from build123d import *

# Parameters (mm, degrees)
BOSS_EXTRUDE1_DEPTH = 1.8
SKETCH2_R           = 3.25
SKETCH2_R_2         = 2.5
BOSS_EXTRUDE3_DEPTH = 0.2
SKETCH5_R           = 3.25
SKETCH5_R_2         = 2
BOSS_EXTRUDE4_DEPTH = 3
CUT_EXTRUDE1_REACH  = 6.8
SKETCH6_R           = 1.5
CUT_EXTRUDE2_REACH  = 6.8
SKETCH8_R           = 0.5


with BuildPart() as part:
    # Sketch1 → Boss-Extrude1 (new body)
    with BuildSketch(Plane.XY):
        with BuildLine():
            Line((1.525163579, 2.869908719), (15.645, 1.543202838))
            ThreePointArc((15.645, 1.543202838), (17.05, 0), (15.645, -1.543202838))
            Line((15.645, -1.543202838), (1.525163579, -2.869908719))
            ThreePointArc((1.525163579, -2.869908719), (-3.25, 0), (1.525163579, 2.869908719))
        make_face()
    extrude(amount=BOSS_EXTRUDE1_DEPTH)

    # Sketch2 → Boss-Extrude3 (add)
    with BuildSketch(Plane.XY):
        Circle(SKETCH2_R)
        Circle(SKETCH2_R_2, mode=Mode.SUBTRACT)
    extrude(amount=-BOSS_EXTRUDE3_DEPTH)

    # Sketch5 → Boss-Extrude4 (add)
    with BuildSketch(Plane.XY.offset(1.8)):
        Circle(SKETCH5_R)
        Circle(SKETCH5_R_2, mode=Mode.SUBTRACT)
    extrude(amount=BOSS_EXTRUDE4_DEPTH)

    # Sketch6 → Cut-Extrude1 (cut, up to next)
    with BuildSketch(Plane.XY, mode=Mode.PRIVATE) as cut_extrude1_sk1:
        Circle(SKETCH6_R)
    cut_extrude1_tool1 = extrude(cut_extrude1_sk1.sketch, amount=CUT_EXTRUDE1_REACH, mode=Mode.PRIVATE) & part.part
    add(cut_extrude1_tool1.solids().sort_by_distance((0, 0, 0))[0], mode=Mode.SUBTRACT)

    # Sketch8 → Cut-Extrude2 (cut, up to next)
    with BuildSketch(Plane.XY, mode=Mode.PRIVATE) as cut_extrude2_sk1:
        with Locations((15.5, 0)):
            Circle(SKETCH8_R)
    cut_extrude2_tool1 = extrude(cut_extrude2_sk1.sketch, amount=CUT_EXTRUDE2_REACH, mode=Mode.PRIVATE) & part.part
    add(cut_extrude2_tool1.solids().sort_by_distance((15.5, 0, 0))[0], mode=Mode.SUBTRACT)
    # Sketch8 → Cut-Extrude2 (cut, up to next)
    with BuildSketch(Plane.XY, mode=Mode.PRIVATE) as cut_extrude2_sk2:
        with Locations((13.3, 0)):
            Circle(SKETCH8_R)
    cut_extrude2_tool2 = extrude(cut_extrude2_sk2.sketch, amount=CUT_EXTRUDE2_REACH, mode=Mode.PRIVATE) & part.part
    add(cut_extrude2_tool2.solids().sort_by_distance((13.3, 0, 0))[0], mode=Mode.SUBTRACT)
    # Sketch8 → Cut-Extrude2 (cut, up to next)
    with BuildSketch(Plane.XY, mode=Mode.PRIVATE) as cut_extrude2_sk3:
        with Locations((11.1, 0)):
            Circle(SKETCH8_R)
    cut_extrude2_tool3 = extrude(cut_extrude2_sk3.sketch, amount=CUT_EXTRUDE2_REACH, mode=Mode.PRIVATE) & part.part
    add(cut_extrude2_tool3.solids().sort_by_distance((11.1, 0, 0))[0], mode=Mode.SUBTRACT)
    # Sketch8 → Cut-Extrude2 (cut, up to next)
    with BuildSketch(Plane.XY, mode=Mode.PRIVATE) as cut_extrude2_sk4:
        with Locations((8.9, 0)):
            Circle(SKETCH8_R)
    cut_extrude2_tool4 = extrude(cut_extrude2_sk4.sketch, amount=CUT_EXTRUDE2_REACH, mode=Mode.PRIVATE) & part.part
    add(cut_extrude2_tool4.solids().sort_by_distance((8.9, 0, 0))[0], mode=Mode.SUBTRACT)
    # Sketch8 → Cut-Extrude2 (cut, up to next)
    with BuildSketch(Plane.XY, mode=Mode.PRIVATE) as cut_extrude2_sk5:
        with Locations((6.7, 0)):
            Circle(SKETCH8_R)
    cut_extrude2_tool5 = extrude(cut_extrude2_sk5.sketch, amount=CUT_EXTRUDE2_REACH, mode=Mode.PRIVATE) & part.part
    add(cut_extrude2_tool5.solids().sort_by_distance((6.7, 0, 0))[0], mode=Mode.SUBTRACT)
    # Sketch8 → Cut-Extrude2 (cut, up to next)
    with BuildSketch(Plane.XY, mode=Mode.PRIVATE) as cut_extrude2_sk6:
        with Locations((4.5, 0)):
            Circle(SKETCH8_R)
    cut_extrude2_tool6 = extrude(cut_extrude2_sk6.sketch, amount=CUT_EXTRUDE2_REACH, mode=Mode.PRIVATE) & part.part
    add(cut_extrude2_tool6.solids().sort_by_distance((4.5, 0, 0))[0], mode=Mode.SUBTRACT)


solid = part.part
Build history of the part. All positions in model axes, mm. A direction names the side the tool comes from. Coordinates: 2 decimals unless noted, no trailing zeros. Order: outer loops, then holes, each group sorted by start corner. A loop starts at its lowest first (then second) coordinate and runs counter-clockwise, first axis right, second up. Notation, with made-up numbers: (40.5, 44) - (86.5, 44) arc R24 ccw to (86.5, 70) - close; hole circle Ø6 at (77.25, 82). An arc over 180 degrees is marked (long way). Write item = value, one per line. Start each with the question number.
1) Saw through at D-D on z = 2.45. Write the cut outline in (x, y), then the cut area to 3 significant figures.
2) Flat gauge pins, fed straight in: pin 1 Ø3 at (x, z) = (2.5, 2) entering from +Y; pin 2 Ø3 at (x, y) = (9, -1) entering from +Z; pin 3 Ø3 at (x, z) = (10, 2.5) entering from -Y. Where does each tip first touch, or does it go through?
3) Saw through at C-C on y = 0. Count the separate pieces of the cut face and the enclosed holes in it, then the cut area to 3 significant figures.
4) 3-axis set-ups, long thin cutter, end or side, ignore diameter. For faces 4 (the face through (-2, 0, 0)), 5 (the face through (0, -2, 3)), 6 (the face through (2, -2, -0.2)): which of +Z, -Z, +X, -X, +Y, -Y reach the whole face in a straight line?
5) Saw through at A-A on x = 0. Write the cut outline in (y, z), then the cut area to 3 significant figures.
6) Two-plate mould, pull along X, no slides. Class faces 1 (the face through (9, 1, 0)), 2 (the face through (17.05, 0.03, 0.89)), 3 (the face through (6.2, 0, 0.9)): pulls with the +X half, pulls with the -X half, needs draft (parallel to the pull), parting line crosses it, or undercut.
7) Saw through at B-B on z = 0.6. Write the cut outline in (x, y) (3 decimals), then the cut area to 3 significant figures.
8) Wall check: line 1 along Y through (x, z) = (0, -0.1); line 2 along X through (y, z) = (1.75, 3.8); line 3 along Y through (x, z) = (-1.5, 2.45). Give the ranges that are in metal, low to high. Write a range as from..to.
From the geometry:
q1.outline = circle Ø6.5 at (0, 0); hole circle Ø4 at (0, 0)
q1.area = 20.6 mm^2
q2.pin_1 = 3.09
q2.pin_2 = 1.8
q2.pin_3 = -2.2
q3.separate_pieces = 8
q3.enclosed_holes = 0
q3.area = 28.1 mm^2
q4.face_4 = -Z
q4.face_5 = +Z
q4.face_6 = -Z, +X, -X, +Y, -Y
q5.outline = (-3.25, -0.2) - (-2.5, -0.2) - (-2.5, 0) - (-1.5, 0) - (-1.5, 1.8) - (-2, 1.8) - (-2, 4.8) - (-3.25, 4.8) - close; (1.5, 0) - (2.5, 0) - (2.5, -0.2) - (3.25, -0.2) - (3.25, 4.8) - (2, 4.8) - (2, 1.8) - (1.5, 1.8) - close
q5.area = 14.1 mm^2
q6.face_1 = needs draft
q6.face_2 = pulls with the +X half
q6.face_3 = undercut
q7.outline = (1.525, -2.87) - (15.645, -1.543) arc R1.55 ccw to (15.645, 1.543) - (1.525, 2.87) arc R3.25 ccw (long way) to start; hole circle Ø3 at (0, 0); hole circle Ø1 at (4.5, 0); hole circle Ø1 at (6.7, 0); hole circle Ø1 at (8.9, 0); hole circle Ø1 at (11.1, 0); hole circle Ø1 at (13.3, 0); hole circle Ø1 at (15.5, 0)
q7.area = 80.0 mm^2
q8.line_1 = -3.25..-2.5, 2.5..3.25
q8.line_2 = -2.74..-0.97, 0.97..2.74
q8.line_3 = -2.88..-1.32, 1.32..2.88
